Input: part model. Units: mm. Frame: model coordinates. Face numbers are marked on the shaded views. A direction names the side the tool comes from. Round coordinates to 2 decimals unless told otherwise and drop trailing zeros. Order: outer loops, then holes, each group sorted by start corner. A loop starts at its lowest first (then second) coordinate and runs counter-clockwise, first axis right, second up.
Item 1: Cut plane A-A on z = 0. Output: boundary loops of the cut face in (x, y), then the cut area to 3 significant figures.
Item 2: Reachability of the marked faces 1, 2 and 3 from +Z, -Z, +X, -X, +Y, -Y: full face, straight path, thin tool, end or side. Return the list, or none.
Item 3: Cut plane C-C on x = 9. Output: boundary loops of the cut face in (y, z), then the cut area to 3 significant figures.
Item 4: First-contact query: pin 1 (1 mm diameter, centred on x = 16.5, y = 5.5, fed in from -Z); pin 2 (3 mm diameter, centred on x = 8.5, z = -6.5, fed in from -Y); pin 3 (1.5 mm diameter, centred on x = 28, z = 0, fed in from -Y). Flat tips, straight axial feed; report the tip coordinate or a pass-through.
Item 5: Line query: L1, parallel to X at y = 4.25, z = -5.5; L2, parallel to Z at x = 39.5, y = 0.5; L3, parallel to Y at x = 2, z = -1.5. Output: solid intervals per line, ascending.
Item 6: Cut plane B-B on x = 37.5. Output: boundary loops of the cut face in (y, z), then the cut area to 3 significant figures.
```python
from build123d import *

# Parameters (mm, degrees)
BOSS_EXTRUDE1_DEPTH         = 10.94232
F_1_4_CLEARANCE_HOLE1_D     = 7.112
F_1_4_CLEARANCE_HOLE1_DEPTH = 15.10284
F_1_4_CLEARANCE_HOLE2_D     = 7.112
F_1_4_CLEARANCE_HOLE2_DEPTH = 15.10284
CHAMFER1_SIZE2              = 1.076433961
CHAMFER1_SIZE               = 1.042413957
CHAMFER1_EDGE_2_SIZE2       = 1.042413957
CHAMFER1_EDGE_2_SIZE        = 1.076433961


with BuildPart() as part:
    # Sketch1 → Boss-Extrude1 (new body)
    with BuildSketch(Plane(origin=(15.10284, 0, 0), x_dir=(0, -1, 0), z_dir=(-1, 0, 0))):
        Polygon((7.14375, -4.124445986), (7.14375, 4.124445986), (0, 8.248891971), (-7.14375, 4.124445986), (-7.14375, -4.124445986), (0, -8.248891971), align=None)
    extrude(amount=-BOSS_EXTRUDE1_DEPTH)

    # Sketch2 → Revolve1 (revolve)
    with BuildSketch(Plane(origin=(0, 0, 0), x_dir=(-1, 0, 0), z_dir=(0, 0, -1))):
        Polygon((-41.148, 6.540243957), (-41.148, 0), (-26.04516, 0), (-26.04516, 6.858), (-30.94228, 6.858), align=None)
    revolve(axis=Axis((41.148, 0, 0), (-1, 0, 0)))

    # Sketch3 → Revolve2 (revolve)
    with BuildSketch(Plane(origin=(0, 0, 0), x_dir=(-1, 0, 0), z_dir=(0, 0, -1))):
        Polygon((-15.10284, 6.858), (-15.10284, 0), (0, 0), (0, 6.540243957), (-10.20572, 6.858), align=None)
    revolve(axis=Axis((15.10284, 0, 0), (-1, 0, 0)))

    # 1/4 Clearance Hole1
    with Locations(Plane(origin=(41.148, 0, 0), x_dir=(0, 0, -1), z_dir=(1, 0, 0))):
        with Locations((0, 0)):
            Hole(F_1_4_CLEARANCE_HOLE1_D / 2, depth=F_1_4_CLEARANCE_HOLE1_DEPTH)

    # 1/4 Clearance Hole2
    with Locations(Plane.ZY):
        with Locations((0, 0)):
            Hole(F_1_4_CLEARANCE_HOLE2_D / 2, depth=F_1_4_CLEARANCE_HOLE2_DEPTH)

    # Chamfer1
    chamfer1_edges = [part.edges().sort_by_distance(p)[0] for p in [
        (41.148, -6.540243957, 0),
    ]]
    chamfer(chamfer1_edges, length=CHAMFER1_SIZE, length2=CHAMFER1_SIZE2)

    # Chamfer1 edge 2
    chamfer1_edge_2_edges = [part.edges().sort_by_distance(p)[0] for p in [
        (0, -6.540243957, 0),
    ]]
    chamfer(chamfer1_edge_2_edges, length=CHAMFER1_EDGE_2_SIZE, length2=CHAMFER1_EDGE_2_SIZE2)


solid = part.part
```
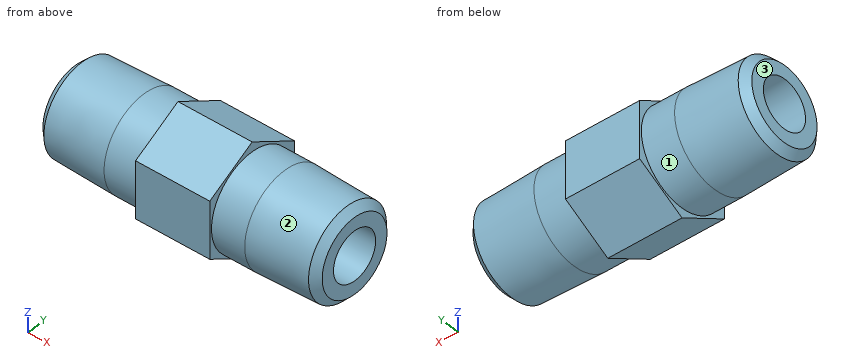
From the geometry:
1. outline: (0, -5.5) - (1.08, -6.57) - (10.21, -6.86) - (15.1, -6.86) - (15.1, -7.14) - (26.05, -7.14) - (26.05, -6.86) - (30.94, -6.86) - (40.11, -6.57) - (41.15, -5.46) - (41.15, -3.56) - (26.05, -3.56) - (26.05, 3.56) - (41.15, 3.56) - (41.15, 5.46) - (40.11, 6.57) - (30.94, 6.86) - (26.05, 6.86) - (26.05, 7.14) - (15.1, 7.14) - (15.1, 6.86) - (10.21, 6.86) - (1.08, 6.57) - (0, 5.5) - (0, 3.56) - (15.1, 3.56) - (15.1, -3.56) - (0, -3.56) - close
1. area: 347 mm2
2. face 1: -X
2. face 2: +X
2. face 3: +Z, -Z, -X, +Y, -Y
3. outline: circle Ø13.64 at (0, 0); hole circle Ø7.11 at (0, 0)
3. area: 106 mm2
4. pin 1: stops at z = -5.36
4. pin 2: stops at y = -4.62
4. pin 3: stops at y = -6.86
5. L1: x = 15.1 to 26.05
5. L2: z = -6.57 to -3.52, 3.52 to 6.57
5. L3: y = -6.43 to -3.22, 3.22 to 6.43
6. outline: circle Ø13.31 at (0, 0); hole circle Ø7.11 at (0, 0)
6. area: 99.4 mm2
